Build history of the part. All positions in model axes, mm. Face numbers are marked on the shaded views. Give positions to 0.01 mm unless a question says otherwise; leave off trailing zeros. Write each loop counter-clockwise with the first axis right and the second up, starting at its lowest first coordinate (ties: lowest second). Pieces come first, ordered by that corner, then holes. Notation, with made-up numbers: (41.5, 8.5) -> (46.5, 8.5) arc R20 cw to (46.5, 24.5) -> close; hole circle Ø7 at (-34.75, -19). An arc over 180 degrees is marked (long way). One line per question, with ' | ' between items. Start each with the question number.
(1) Band-saw the part on B-B, the plane x = 16.5. Give the cut face in (y, z), and give its area (3 significant figures).
(2) Pull direction Y, two halves, no side cores. Call the marked faces 1 and 2: released by +Y, released by -Y, zero draft, split by the parting line, or undercut.
(3) Pin check, flat tips, straight feed: P1, Ø1.4, axis at x = 46.5, y = 22.5, coming from the -Z side; P2, Ø10.5, axis at x = 33.239, y = 8, coming from the -Z side. Stop position of each tip, or through.
(4) Drill centre lines: probe 1 along X at (y, z) = (11.5, 0.5); probe 2 along Y at (x, z) = (19, 0.75); probe 3 along X at (y, z) = (22.5, 1). Where is each one in solid material? Low to high. Write a range as from..to.
(5) Band-saw the part on A-A, the plane z = -2.75. Give the cut face in (x, y).
from build123d import *

# Parameters (mm, degrees)
SKETCH2_R           = 1.8
SKETCH2_R_2         = 3.6
SKETCH2_R_3         = 4
SKETCH2_R_4         = 1.45
SKETCH2_R_5         = 1.85
SKETCH2_W           = 28.1
SKETCH2_H           = 8.2
BOSS_EXTRUDE2_DEPTH = 1.5
SKETCH3_R           = 2.4
SKETCH3_R_2         = 0.9
BOSS_EXTRUDE3_DEPTH = 1.6
SKETCH4_R           = 2.4
SKETCH4_R_2         = 0.9
BOSS_EXTRUDE4_DEPTH = 4.8
CHAMFER1_SIZE       = 0.5


with BuildPart() as part:
    # Sketch2 → Boss-Extrude2 (new body)
    with BuildSketch(Plane.XY):
        with BuildLine():
            Line((0, 22.989), (0, 3.935))
            ThreePointArc((0, 3.935), (1.152534816, 1.152534816), (3.935, 0))
            Line((3.935, 0), (74.043, 0))
            ThreePointArc((74.043, 0), (76.825465184, 1.152534816), (77.978, 3.935))
            Line((77.978, 3.935), (77.978, 22.989))
            ThreePointArc((77.978, 22.989), (76.825465184, 25.771465184), (74.043, 26.924))
            Line((74.043, 26.924), (3.935, 26.924))
            ThreePointArc((3.935, 26.924), (1.152534816, 25.771465184), (0, 22.989))
        make_face()
        with Locations((3.989, 22.962)):
            Circle(SKETCH2_R, mode=Mode.SUBTRACT)
        with Locations((73.989, 22.962)):
            Circle(SKETCH2_R, mode=Mode.SUBTRACT)
        with Locations((3.989, 3.962)):
            Circle(SKETCH2_R, mode=Mode.SUBTRACT)
        with Locations((73.989, 3.962)):
            Circle(SKETCH2_R, mode=Mode.SUBTRACT)
        with Locations((55.978, 13.462)):
            Circle(SKETCH2_R_2, mode=Mode.SUBTRACT)
        with Locations((13.239, 8)):
            Circle(SKETCH2_R_3, mode=Mode.SUBTRACT)
        with Locations((33.239, 8)):
            Circle(SKETCH2_R_3, mode=Mode.SUBTRACT)
        with Locations((41.289, 21.574)):
            Circle(SKETCH2_R_4, mode=Mode.SUBTRACT)
        with Locations((41.289, 17.574)):
            Circle(SKETCH2_R_4, mode=Mode.SUBTRACT)
        with Locations((69.978, 13.462)):
            Circle(SKETCH2_R_5, mode=Mode.SUBTRACT)
        with Locations((23.239, 19.574)):
            Rectangle(SKETCH2_W, SKETCH2_H, mode=Mode.SUBTRACT)
    extrude(amount=BOSS_EXTRUDE2_DEPTH)

    # Sketch3 → Boss-Extrude3 (add)
    # profile 1 of 2: a face of its own
    with BuildSketch(Plane(origin=(0, 0, 0), x_dir=(-1, 0, 0), z_dir=(0, 0, -1))):
        with Locations(Location((-46.239, 22.674, 0), (0, 0, 180))):
            Circle(SKETCH3_R)
        with Locations((-46.239, 22.674)):
            Circle(SKETCH3_R_2, mode=Mode.SUBTRACT)
    # profile 2 of 2: a face of its own
    with BuildSketch(Plane(origin=(0, 0, 0), x_dir=(-1, 0, 0), z_dir=(0, 0, -1))):
        with BuildLine():
            Line((-9.189, 15.474), (-9.670742423, 15.474))
            ThreePointArc((-9.670742423, 15.474), (-5.126472799, 16.051548555), (-9.189, 18.168107435))
            Line((-9.189, 18.168107435), (-9.189, 15.474))
        make_face()
        with Locations((-7.489, 16.474)):
            Circle(SKETCH3_R_2, mode=Mode.SUBTRACT)
    extrude(amount=BOSS_EXTRUDE3_DEPTH)

    # Sketch4 → Boss-Extrude4 (add)
    # profile 1 of 3: a face of its own
    with BuildSketch(Plane(origin=(0, 0, 0), x_dir=(-1, 0, 0), z_dir=(0, 0, -1))):
        with Locations(Location((-67.228, 20.962, 0), (0, 0, 180))):
            Circle(SKETCH4_R)
        with Locations((-67.228, 20.962)):
            Circle(SKETCH4_R_2, mode=Mode.SUBTRACT)
    # profile 2 of 3: a face of its own
    with BuildSketch(Plane(origin=(0, 0, 0), x_dir=(-1, 0, 0), z_dir=(0, 0, -1))):
        with Locations(Location((-67.228, 5.962, 0), (0, 0, 180))):
            Circle(SKETCH4_R)
        with Locations((-67.228, 5.962)):
            Circle(SKETCH4_R_2, mode=Mode.SUBTRACT)
    # profile 3 of 3: a face of its own
    with BuildSketch(Plane(origin=(0, 0, 0), x_dir=(-1, 0, 0), z_dir=(0, 0, -1))):
        with Locations(Location((-45.728, 5.962, 0), (0, 0, 180))):
            Circle(SKETCH4_R)
        with Locations((-45.728, 5.962)):
            Circle(SKETCH4_R_2, mode=Mode.SUBTRACT)
    extrude(amount=BOSS_EXTRUDE4_DEPTH)

    # Chamfer1
    chamfer1_edges = [part.edges().sort_by_distance(p)[0] for p in [
        (5.126472799, 16.051548555, 0),
        (43.839, 22.674, 0),
        (64.828, 20.962, 0),
        (64.828, 5.962, 0),
        (43.328, 5.962, 0),
    ]]
    chamfer(chamfer1_edges, length=CHAMFER1_SIZE)


solid = part.part
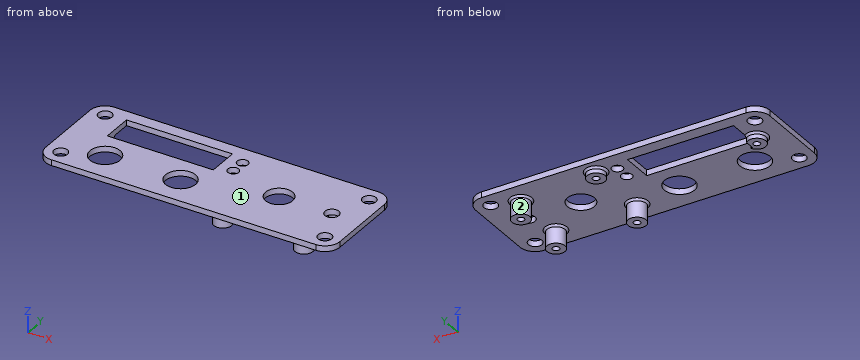
Results:
1) outline: (0, 0) -> (5.68, 0) -> (5.68, 1.5) -> (0, 1.5) -> close; (10.32, 0) -> (15.47, 0) -> (15.47, 1.5) -> (10.32, 1.5) -> close; (23.67, 0) -> (26.92, 0) -> (26.92, 1.5) -> (23.67, 1.5) -> close | area: 21.1 mm²
2) face 1: zero draft | face 2: undercut
3) P1: stops at z = -1.6 | P2: stops at z = 0
4) probe 1: x = 0..11.3, 15.18..31.3, 35.18..52.96, 59..77.98 | probe 2: y = 0..15.47, 23.67..26.92 | probe 3: x = 0..2.25, 5.73..9.19, 37.29..40.17, 42.4..72.25, 75.73..77.98
5) outline: circle Ø4.8 at (45.73, 5.96); circle Ø4.8 at (67.23, 5.96); circle Ø4.8 at (67.23, 20.96); hole circle Ø1.8 at (45.73, 5.96); hole circle Ø1.8 at (67.23, 5.96); hole circle Ø1.8 at (67.23, 20.96)
